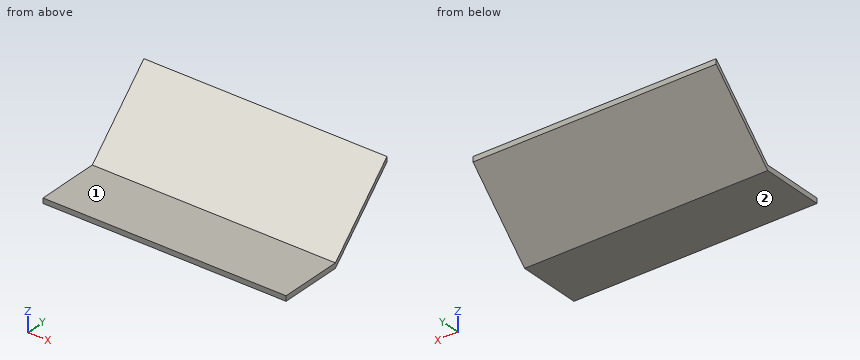
Autodesk Inventor part; units mm, degrees
ref_plane "YZ Plane" through (0, 0, 0) normal (1, 0, 0) x (0, 1, 0)
ref_plane "XZ Plane" through (0, 0, 0) normal (0, 1, 0) x (-1, 0, 0)
ref_plane "XY Plane" through (0, 0, 0) normal (0, 0, 1) x (1, 0, 0)
sketch "Esboço1" plane through (0, 0, 0) normal (1, 0, 0) x (0, 1, 0)
  line L0 (30.2603, -55.8743) -> (4.9294, -55.8743)
  line L1 (30.2603, -57.9073) -> (4.9294, -57.9073)
  line L2 (56.7603, -29.3743) -> (30.2603, -55.8743)
  line L3 (56.7603, -31.3743) -> (30.2603, -57.9073)
  line L4 (4.9294, -55.8743) -> (4.9294, -57.9073)
  line L5 (56.7603, -29.3743) -> (56.7603, -31.3743)
  point P0 (0, 0)
  point P1 (56.7603, -55.8743)
  point P2 (56.7603, -55.8743)
  dimension "d4" = 26.5
  dimension "d5" = 26.5
  dimension "d6" = 2
  dimension "d7" = 37.5
extrude "Extrusão1" add sketch "Esboço1" along normal blind 97
properties part number "Mini Sumô Definitivo - TAMPA"
Verification items for the finished model (mm, model axes). Face numbers are marked on the shaded views. A direction names the side the tool comes from. Coordinates: 2 decimals unless noted, no trailing zeros. Write each loop counter-clockwise with the first axis right and the second up, starting at its lowest first coordinate (ties: lowest second). Pieces come first, ordered by that corner, then holes. Notation, with made-up numbers: M 48,-18 L 81,-18 A20 cw 81,2 Z; hole C 51,78.5 d1. An arc over 180 degrees is marked long. One line per question, with ' | ' between items.
1) Material ranges on L1, parallel to Z at x = 86, y = 23; L2, parallel to Y at x = 30, z = -44; L3, parallel to Y at x = 50, z = -53.5, recorded low to high.
Solutions:
L1: -57.91 to -55.87 | L2: 42.13 to 44.15 | L3: 32.63 to 34.66
2) Sectioned sample at C-C on z = -52.5. Record the cut outline in (x, y), then the cut area to 3 significant figures.
Solutions:
outline: M 0,33.63 L 97,33.63 L 97,35.66 L 0,35.66 Z | area: 197 mm^2
3) Depth check by flat-ended pin: pin 1 Ø6 at (x, z) = (32.5, -47.5) entering from -Y; pin 2 Ø1 at (x, y) = (55, 46) entering from +Z; pin 3 Ø1 at (x, z) = (51, -50.5) entering from -Y; pin 4 Ø6 at (y, z) = (39.5, -39) entering from -X. Enter the tip coordinate at first touch or a pass-through.
Solutions:
pin 1: y = 35.63 | pin 2: z = -39.63 | pin 3: y = 35.13 | pin 4: through
4) Access from +Z, -Z, +X, -X, +Y, -Y to the whole of each face (thin tool, end or side, straight path). Record for the marked faces 1 and 2.
Solutions:
face 1: +Z, +X, -X, -Y | face 2: -Z, +X, -X, +Y, -Y
5) Sectioned sample at B-B on y = 27.5. Record the cut outline in (x, z).
Solutions:
outline: M 0,-57.91 L 97,-57.91 L 97,-55.87 L 0,-55.87 Z
6) Sectioned sample at A-A on x = 7. Record the cut outline in (y, z), then the cut area to 3 significant figures.
Solutions:
outline: M 4.93,-57.91 L 30.26,-57.91 L 56.76,-31.37 L 56.76,-29.37 L 30.26,-55.87 L 4.93,-55.87 Z | area: 105 mm^2
